Answer from the drawing. Dimensions are ordinates in mm from the lowest x, y and z of the part. Round coordinates to 2 decimals unless told otherwise and drop trailing zeros. Order: outer loops, then holes, each group sorted by start corner. A loop starts at its lowest first (then second) coordinate and runs counter-clockwise, first axis right, second up. Notation, with made-up numbers: (68, -36) -> (104, -36) arc R20 cw to (104, -22) -> close; hole circle Ø4 at (42, 61). An arc over 180 degrees is marked (long way). Use a Markdown table: item, result. Add a question column.
Item 1: A cutting plane is placed at A-A, the plane z = 20.45. Determine the outline of the cut face in (x, y) (3 decimals), plus the area to 4 significant figures.
Item 2: A cutting plane is placed at D-D, the plane x = 9. Determine the outline of the cut face in (y, z).
Item 3: Find the intervals of material crossed by L1, parallel to X at y = 0.35, z = 20.45 (3 decimals); L2, parallel to Y at x = 36, z = 59; L3, parallel to X at y = 3.6, z = 4.5, in increasing order. Write a range as [from, to].
Item 4: A flat-ended cylindrical pin translates along its axis: P1, Ø1, axis at x = 34, z = 17, coming from the +Y side. Find the tip coordinate at first contact, or state that the pin passes through.
Item 5: A cutting plane is placed at C-C, the plane z = 47.33. Determine the outline of the cut face in (x, y) (3 decimals).
Item 6: A cutting plane is placed at B-B, the plane y = 2.05. Determine the outline of the cut face in (x, z) (3 decimals), plus the area to 3 significant figures.
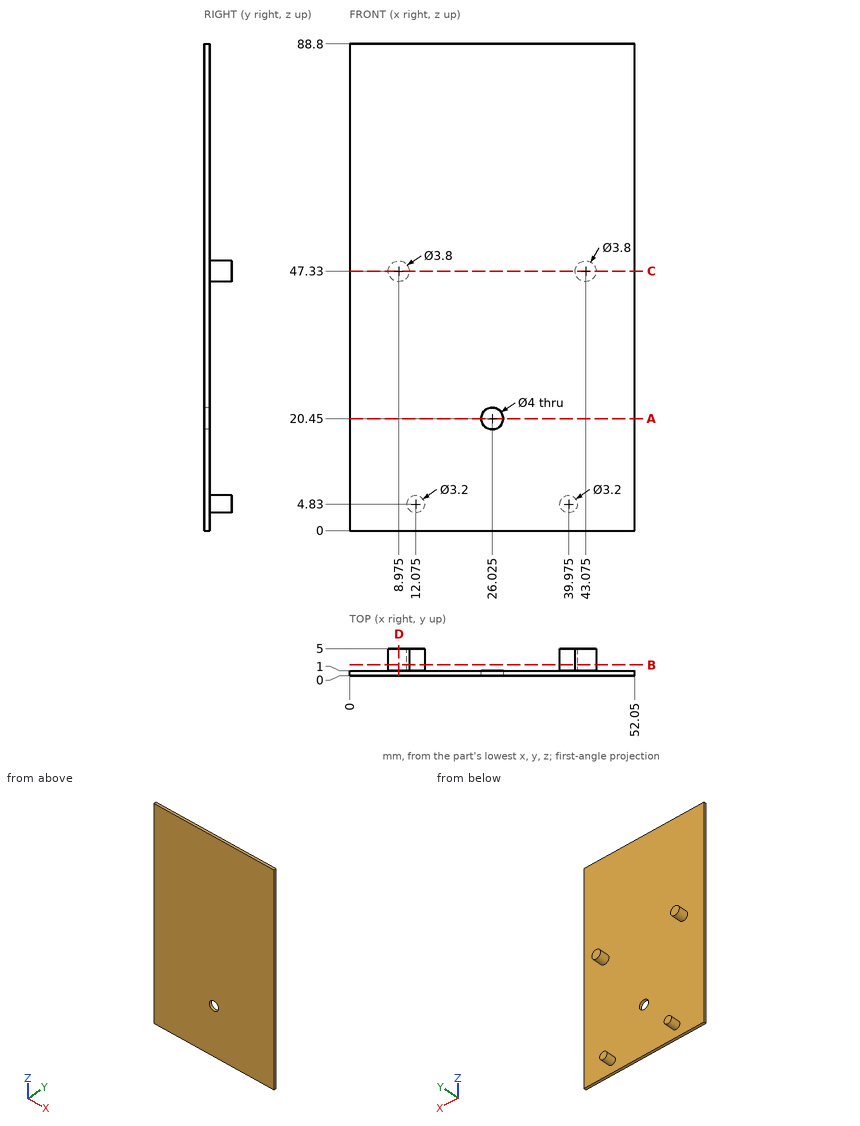
Reported:
| question | item | result |
|---|---|---|
| 1 | outline | (0, 0) -> (24.025, 0) -> (24.025, 1) -> (0, 1) -> close; (28.025, 0) -> (52.05, 0) -> (52.05, 1) -> (28.025, 1) -> close |
| 1 | area | 48.05 mm² |
| 2 | outline | (0, 0) -> (1, 0) -> (1, 45.43) -> (5, 45.43) -> (5, 49.23) -> (1, 49.23) -> (1, 88.8) -> (0, 88.8) -> close |
| 3 | L1 | [0, 24.025], [28.025, 52.05] |
| 3 | L2 | [0, 1] |
| 3 | L3 | [10.51, 13.64], [38.41, 41.54] |
| 4 | P1 | y = 1 |
| 5 | outline | (0, 0) -> (52.05, 0) -> (52.05, 1) -> (44.975, 1) -> (44.975, 5) -> (41.175, 5) -> (41.175, 1) -> (10.875, 1) -> (10.875, 5) -> (7.075, 5) -> (7.075, 1) -> (0, 1) -> close |
| 6 | outline | circle Ø3.8 at (8.975, 47.33); circle Ø3.2 at (12.075, 4.83); circle Ø3.2 at (39.975, 4.83); circle Ø3.8 at (43.075, 47.33) |
| 6 | area | 38.8 mm² |
